For this review, take the finished solid that the model builds, in its own axes (mm). A direction names the side the tool comes from. Round coordinates to 2 decimals unless told otherwise and drop trailing zeros. Loops run counter-clockwise (first coordinate to the right, second up) from the corner with the lowest first, then second, coordinate; pieces in that order, holes last. Notation, with made-up numbers: M 45,86 L 99,86 A16 cw 99,100 Z; hole C -33,7 d9. An arc over 180 degrees is marked long. Write item = value, one per line. Start each with the question number.
```python
from build123d import *

# Parameters (mm, degrees)
F0_W     = 94
F0_H     = 4
F1_DEPTH = 4
F3_DEPTH = 5
F4_DEPTH = 1


with BuildPart() as f1:
    # F0 (on Top) → F1 (new body)
    with BuildSketch(Plane.XY):
        with BuildLine():
            ThreePointArc((2.426764, 2.23625), (0, -3.3), (-2.426764, 2.23625))
            ThreePointArc((-2.426764, 2.23625), (-2.699268, 2.69082), (-2.887527, 3.18625))
            ThreePointArc((-2.887527, 3.18625), (-4.299127, -0.08664), (-2.75681, -3.3))
            Line((-2.75681, -3.3), (-2.75681, -7.3))
            Line((-2.75681, -7.3), (2.75681, -7.3))
            Line((2.75681, -7.3), (2.75681, -3.3))
            ThreePointArc((2.75681, -3.3), (4.299127, -0.08664), (2.887527, 3.18625))
            ThreePointArc((2.887527, 3.18625), (2.699268, 2.69082), (2.426764, 2.23625))
        make_face()
        with Locations((-49.75681, -5.3)):
            Rectangle(F0_W, F0_H)
    extrude(amount=F1_DEPTH)

    # F2 (on face) → F3 (join)
    with BuildSketch(Plane.XZ.offset(7.3)):
        with BuildLine():
            ThreePointArc((-91.573236, 9.53625), (-94, 4), (-96.426764, 9.53625))
            ThreePointArc((-96.426764, 9.53625), (-96.699268, 9.99082), (-96.887527, 10.48625))
            ThreePointArc((-96.887527, 10.48625), (-98.299127, 7.21336), (-96.75681, 4))
            Line((-96.75681, 4), (-96.75681, 1))
            Line((-96.75681, 1), (-91.24319, 1))
            Line((-91.24319, 1), (-91.24319, 4))
            ThreePointArc((-91.24319, 4), (-89.700873, 7.21336), (-91.112473, 10.48625))
            ThreePointArc((-91.112473, 10.48625), (-91.300732, 9.99082), (-91.573236, 9.53625))
        make_face()
    extrude(amount=-F3_DEPTH)

    # F2 (on face) → F4 (join)
    with BuildSketch(Plane.XZ.offset(7.3)):
        with BuildLine():
            ThreePointArc((-91.573236, 9.53625), (-94, 4), (-96.426764, 9.53625))
            ThreePointArc((-96.426764, 9.53625), (-96.699268, 9.99082), (-96.887527, 10.48625))
            ThreePointArc((-96.887527, 10.48625), (-98.299127, 7.21336), (-96.75681, 4))
            Line((-96.75681, 4), (-96.75681, 1))
            Line((-96.75681, 1), (-91.24319, 1))
            Line((-91.24319, 1), (-91.24319, 4))
            ThreePointArc((-91.24319, 4), (-89.700873, 7.21336), (-91.112473, 10.48625))
            ThreePointArc((-91.112473, 10.48625), (-91.300732, 9.99082), (-91.573236, 9.53625))
        make_face()
    extrude(amount=F4_DEPTH)


solid = f1.part
```
(1) Tool access review of faces 1 (the flat face through (2.757, -5, 2)), 2 (the flat face through (-94, -8.3, 3.7)): name each direction out of +Z, -Z, +X, -X, +Y, -Y from which nothing blocks a thin tool from reaching the whole face with its end or side.
(2) Add section A-A on y = 0. Write out the cut boundary in (x, z), and give its area (3 significant figures).
(3) Add section C-C on x = -94. Write out the cut boundary in (y, z), and give its area (3 significant figures).
(4) Wall thickness on L1, parallel to X at y = 0, z = 2.75; L2, parallel to X at y = -5.75, z = 7.3; L3, parallel to Z at x = -94, y = -6.75: over which ranges is each line inside the solid? List them lowest first.
(5) Draft analysis for pull direction Y (two halves, no side actions). For faces 3 (the cylindrical face through (0.1, -3.3, 2)), 4 (the flat face through (-96.757, -5, 2)), 5 (the flat face through (-94, -2.3, 3.7)), state which applies: +Y half, -Y half, draft (parallel to the pull), parting line (faces both ways), or undercut.
(6) For pin 1 Ø2 at (y, z) = (-5, 2) entering from +X; pin 2 Ø4.5 at (x, z) = (-68, 2.5) entering from -Y; pin 3 Ø0.5 at (y, z) = (-8, 2) entering from +X; pin 4 Ø5.5 at (x, y) = (0, 0) entering from +Z, all flat-tipped, find the tip position at first contact; note any pin that passes through.
(7) Add section B-B on z = 7.3. Write out the cut boundary in (x, y), and give its area (3 significant figures).
(8) Add section D-D on x = -18. Write out the cut boundary in (y, z).
Answer sheet:
q1.face_1 = +Z, -Z, +X, -Y
q1.face_2 = +Z, -Z, +X, -X, -Y
q2.outline = M -4.3,0 L -3.3,0 L -3.3,4 L -4.3,4 Z; M 3.3,0 L 4.3,0 L 4.3,4 L 3.3,4 Z
q2.area = 8.00 mm²
q3.outline = M -8.3,1 L -7.3,1 L -7.3,0 L -3.3,0 L -3.3,1 L -2.3,1 L -2.3,4 L -8.3,4 Z
q3.area = 22.0 mm²
q4.L1 = -4.3 to -3.3, 3.3 to 4.3
q4.L2 = -98.3 to -97.3, -90.7 to -89.7
q4.L3 = 0 to 4
q5.face_3 = undercut
q5.face_4 = draft
q5.face_5 = +Y half
q6.pin_1 = 2.76
q6.pin_2 = -7.3
q6.pin_3 = -91.24
q6.pin_4 = through
q7.outline = M -98.3,-8.3 L -97.3,-8.3 L -97.3,-2.3 L -98.3,-2.3 Z; M -90.7,-8.3 L -89.7,-8.3 L -89.7,-2.3 L -90.7,-2.3 Z
q7.area = 12.0 mm²
q8.outline = M -7.3,0 L -3.3,0 L -3.3,4 L -7.3,4 Z
